Build history of the part. All positions in model axes, mm. Coordinates: 2 decimals unless noted, no trailing zeros. Loops run counter-clockwise (first coordinate to the right, second up) from the corner with the lowest first, then second, coordinate; pieces in that order, holes last.
Item 1: Cut at B-B (x = 0). List the corners of the cut face in (y, z), and give its area (3 significant figures).
Item 2: Cut at D-D (z = -11). List the corners of the cut face in (x, y), and give its area (3 significant figures).
Item 3: Drill centre lines: line 1 along Y through (x, z) = (-28, 1); line 2 along Z through (x, y) = (-25.5, 2.5); line 3 along Y through (x, z) = (28.5, 3.8). Where is each one in solid material? Low to high.
Item 4: Cut at C-C (y = 19.5). List the corners of the cut face in (x, z), and give its area (3 significant figures).
Item 5: Flat gauge pins, fed straight in: pin 1 (5 mm diameter, centred on x = 19.5, z = -64.5, fed in from -Y); pin 2 (6 mm diameter, centred on x = 28.5, y = 0, fed in from +Z); pin 3 (8 mm diameter, centred on x = -8, z = -72.5, fed in from +Y). Where does each tip first touch, or does it go through?
Item 6: Cut at A-A (y = 0). Count the separate pieces of the cut face and the enclosed holes in it, and give its area (3 significant figures).
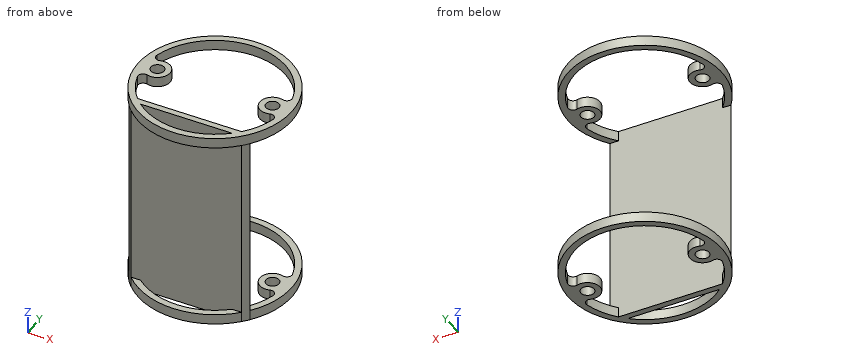
from build123d import *

# Parameters (mm, degrees)
SKETCH1_R           = 38
SKETCH1_R_2         = 3.25
BOSS_EXTRUDE1_DEPTH = 5
BOSS_EXTRUDE2_START = 90
BOSS_EXTRUDE2_DEPTH = 90
BOSS_EXTRUDE3_START = 5
SKETCH3_R           = 3.25
BOSS_EXTRUDE3_DEPTH = 5


with BuildPart() as part:
    # Sketch1 → Boss-Extrude1 (new body)
    with BuildSketch(Plane.XY):
        Circle(SKETCH1_R)
        with Locations((-28.5, 0)):
            Circle(SKETCH1_R_2, mode=Mode.SUBTRACT)
        with Locations((28.5, 0)):
            Circle(SKETCH1_R_2, mode=Mode.SUBTRACT)
        with BuildLine():
            Line((-25.759706908, -23.323807579), (25.759706908, -23.323807579))
            ThreePointArc((25.759706908, -23.323807579), (30.518267855, -16.619200556), (33.568509452, -8.984301485))
            ThreePointArc((33.568509452, -8.984301485), (32.879612131, -6.529477906), (30.395363409, -5.955677757))
            ThreePointArc((30.395363409, -5.955677757), (22.25, 0), (30.395363409, 5.955677757))
            ThreePointArc((30.395363409, 5.955677757), (32.879612131, 6.529477906), (33.568509452, 8.984301485))
            ThreePointArc((33.568509452, 8.984301485), (0, 34.75), (-33.568509452, 8.984301485))
            ThreePointArc((-33.568509452, 8.984301485), (-32.879612131, 6.529477906), (-30.395363409, 5.955677757))
            ThreePointArc((-30.395363409, 5.955677757), (-22.25, 0), (-30.395363409, -5.955677757))
            ThreePointArc((-30.395363409, -5.955677757), (-32.879612131, -6.529477906), (-33.568509452, -8.984301485))
            ThreePointArc((-33.568509452, -8.984301485), (-30.518267855, -16.619200556), (-25.759706908, -23.323807579))
        make_face(mode=Mode.SUBTRACT)
        with BuildLine():
            Line((-22.685229876, -26.323807579), (22.685229876, -26.323807579))
            ThreePointArc((22.685229876, -26.323807579), (0, -34.75), (-22.685229876, -26.323807579))
        make_face(mode=Mode.SUBTRACT)
    extrude(amount=BOSS_EXTRUDE1_DEPTH)

    # Sketch2 → Boss-Extrude2 (add)
    with BuildSketch(Plane(origin=(0, 0, 0), x_dir=(-1, 0, 0), z_dir=(0, 0, -1)).offset(BOSS_EXTRUDE2_START)):
        with BuildLine():
            Line((-30, -23.323807579), (30, -23.323807579))
            ThreePointArc((30, -23.323807579), (28.741879175, -24.857682545), (27.405421991, -26.323807579))
            Line((27.405421991, -26.323807579), (-27.405421991, -26.323807579))
            ThreePointArc((-27.405421991, -26.323807579), (-28.741879175, -24.857682545), (-30, -23.323807579))
        make_face()
    extrude(amount=-BOSS_EXTRUDE2_DEPTH)

    # Sketch3 → Boss-Extrude3 (add)
    with BuildSketch(Plane(origin=(0, 0, -90), x_dir=(-1, 0, 0), z_dir=(0, 0, -1)).offset(BOSS_EXTRUDE3_START)):
        with BuildLine():
            ThreePointArc((-30, -23.323807579), (-28.741879175, -24.857682545), (-27.405421991, -26.323807579))
            ThreePointArc((-27.405421991, -26.323807579), (0, -38), (27.405421991, -26.323807579))
            ThreePointArc((27.405421991, -26.323807579), (28.741879175, -24.857682545), (30, -23.323807579))
            ThreePointArc((30, -23.323807579), (0, 38), (-30, -23.323807579))
        make_face()
        with Locations(Location((28.5, 0, 0), (0, 0, 180))):
            Circle(SKETCH3_R, mode=Mode.SUBTRACT)
        with Locations(Location((-28.5, 0, 0), (0, 0, 180))):
            Circle(SKETCH3_R, mode=Mode.SUBTRACT)
        with BuildLine():
            Line((-22.685229876, -26.323807579), (22.685229876, -26.323807579))
            ThreePointArc((22.685229876, -26.323807579), (0, -34.75), (-22.685229876, -26.323807579))
        make_face(mode=Mode.SUBTRACT)
        with BuildLine():
            Line((25.759706908, -23.323807579), (-25.759706908, -23.323807579))
            ThreePointArc((-25.759706908, -23.323807579), (-30.518267855, -16.619200556), (-33.568509452, -8.984301485))
            ThreePointArc((-33.568509452, -8.984301485), (-32.879612131, -6.529477906), (-30.395363409, -5.955677757))
            ThreePointArc((-30.395363409, -5.955677757), (-22.25, 0), (-30.395363409, 5.955677757))
            ThreePointArc((-30.395363409, 5.955677757), (-32.879612131, 6.529477906), (-33.568509452, 8.984301485))
            ThreePointArc((-33.568509452, 8.984301485), (0, 34.75), (33.568509452, 8.984301485))
            ThreePointArc((33.568509452, 8.984301485), (32.879612131, 6.529477906), (30.395363409, 5.955677757))
            ThreePointArc((30.395363409, 5.955677757), (22.25, 0), (30.395363409, -5.955677757))
            ThreePointArc((30.395363409, -5.955677757), (32.879612131, -6.529477906), (33.568509452, -8.984301485))
            ThreePointArc((33.568509452, -8.984301485), (30.518267855, -16.619200556), (25.759706908, -23.323807579))
        make_face(mode=Mode.SUBTRACT)
    extrude(amount=-BOSS_EXTRUDE3_DEPTH)


solid = part.part
Filled sheet:
1. outline: (-38, -95) - (-34.75, -95) - (-34.75, -90) - (-38, -90) - close; (-38, 0) - (-34.75, 0) - (-34.75, 5) - (-38, 5) - close; (-26.32, -95) - (-23.32, -95) - (-23.32, 5) - (-26.32, 5) - close; (34.75, -95) - (38, -95) - (38, -90) - (34.75, -90) - close; (34.75, 0) - (38, 0) - (38, 5) - (34.75, 5) - close
1. area: 365 mm2
2. outline: (-30, -23.32) arc R38 ccw to (-27.41, -26.32) - (27.41, -26.32) arc R38 ccw to (30, -23.32) - close
2. area: 172 mm2
3. line 1: y = -25.69 to -20.58, -6.23 to -3.21, 3.21 to 6.23, 20.58 to 25.69
3. line 2: z = -95 to -90, 0 to 5
3. line 3: y = -25.13 to -19.88, -6.25 to -3.25, 3.25 to 6.25, 19.88 to 25.13
4. outline: (-32.62, -95) - (-28.76, -95) - (-28.76, -90) - (-32.62, -90) - close; (-32.62, 0) - (-28.76, 0) - (-28.76, 5) - (-32.62, 5) - close; (28.76, -95) - (32.62, -95) - (32.62, -90) - (28.76, -90) - close; (28.76, 0) - (32.62, 0) - (32.62, 5) - (28.76, 5) - close
4. area: 77.0 mm2
5. pin 1: stops at y = -26.32
5. pin 2: passes through
5. pin 3: stops at y = -23.32
6. separate pieces: 8
6. enclosed holes: 0
6. area: 185 mm2
